```python
from build123d import *

# Parameters (mm, degrees)
BOSS_EXTRUDE1_DEPTH = 2.5


with BuildPart() as part:
    # Sketch1 → Boss-Extrude1 (new body)
    with BuildSketch(Plane.XY):
        with BuildLine():
            Line((-6.062552239, 2.5), (-6.062552239, -2.5))
            add(Edge.make_bspline(
                [(-3.378314474, -1.025559537), (-4.49216768, -0.325238314), (-5.082460235, -2.568455815), (-6.062552239, -2.5)],
                knots=[0, 0, 0, 0, 1, 1, 1, 1], degree=3))
            add(Edge.make_bspline(
                [(0, -2.5), (-2.128381344, -2.596064875), (-3.378314474, -1.025559537)],
                knots=[0, 0, 0, 1, 1, 1], degree=2))
            Line((0, -2.5), (0, -2.4))
            ThreePointArc((0, -2.4), (-2.4, 0), (0, 2.4))
            Line((0, 2.4), (0, 2.5))
            add(Edge.make_bspline(
                [(0, 2.5), (-2.128381344, 2.596064875), (-3.378314474, 1.025559537)],
                knots=[0, 0, 0, 1, 1, 1], degree=2))
            add(Edge.make_bspline(
                [(-3.378314474, 1.025559537), (-4.49216768, 0.325238314), (-5.082460235, 2.568455815), (-6.062552239, 2.5)],
                knots=[0, 0, 0, 0, 1, 1, 1, 1], degree=3))
        make_face()
    extrude(amount=BOSS_EXTRUDE1_DEPTH)


solid = part.part
```
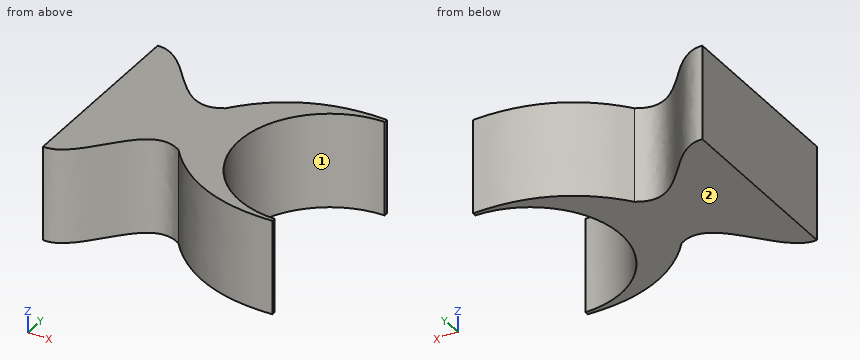
The listing builds one solid part. Answer for the finished solid, in the listing's coordinates (mm). Face numbers are marked on the shaded views. Give positions to 0.01 mm unless a question says otherwise; leave off trailing zeros. Order: outer loops, then holes, each group sorted by start corner. A loop starts at its lowest first (then second) coordinate and runs counter-clockwise, first axis right, second up. Notation, with made-up numbers: (-31, 31.25) -> (-27, 31.25) arc R34 cw to (-27, 64.25) -> close; hole circle Ø9 at (55, -2.75). An arc over 180 degrees is marked (long way). One line per item, written item: value.
1) Find the intervals of material crossed by line 1 (X direction, y = 2.15, z = 2.2); line 2 (X direction, y = -1.15, z = 2.3); line 3 (Y direction, x = -0.5, z = 0.4), in increasing order.
Reported:
line 1: x = -6.06 to -5.33, -1.97 to -1.07
line 2: x = -6.06 to -4.4, -3.28 to -2.11
line 3: y = -2.5 to -2.35, 2.35 to 2.5
2) Find section A-A, the plane y = 0. Determine the outline of the cut face in (x, z).
Reported:
outline: (-6.06, 0) -> (-2.4, 0) -> (-2.4, 2.5) -> (-6.06, 2.5) -> close
3) Determine the mould class of the marked faces 1 and 2 for opening direction Y: pulls with the +Y half, pulls with the -Y half, needs draft (parallel to the pull), parting line crosses it, or undercut.
Reported:
face 1: undercut
face 2: needs draft
